from build123d import *

# Parameters (mm, degrees)
SKETCH1_R           = 6
SKETCH1_W           = 9.664317132
SKETCH1_H           = 5.093827802
BOSS_EXTRUDE1_DEPTH = 58
SKETCH2_R           = 2.5
SKETCH2_R_2         = 1.557642262
CUT_EXTRUDE1_DEPTH  = 10


with BuildPart() as part:
    # Sketch1 → Boss-Extrude1 (new body)
    with BuildSketch(Plane.XY):
        with BuildLine():
            Line((-9.822104082, -25.661413332), (-5.082925118, -30.205025059))
            ThreePointArc((-5.082925118, -30.205025059), (-5.444381805, -30.665269108), (-5.771113852, -31.15078089))
            Line((-5.771113852, -31.15078089), (-9.145384533, -28.943772104))
            Line((-9.145384533, -28.943772104), (-9.823578986, -29.980655904))
            Line((-9.823578986, -29.980655904), (-6.344193142, -32.256417352))
            ThreePointArc((-6.344193142, -32.256417352), (-6.488837019, -32.624364602), (-6.615069482, -32.999027645))
            Line((-6.615069482, -32.999027645), (-9.783580045, -32.250497314))
            Line((-9.783580045, -32.250497314), (-10.034391467, -33.312175922))
            Line((-10.034391467, -33.312175922), (-6.865985046, -34.060689065))
            ThreePointArc((-6.865985046, -34.060689065), (-6.932730681, -34.565893765), (-6.967078624, -35.074329589))
            Line((-6.967078624, -35.074329589), (-9.963607891, -35.148687431))
            Line((-9.963607891, -35.148687431), (-9.93976563, -36.109501168))
            Line((-9.93976563, -36.109501168), (-6.926935836, -36.033753282))
            ThreePointArc((-6.926935836, -36.033753282), (-6.847527662, -36.665356301), (-6.717901152, -37.288593816))
            Line((-6.717901152, -37.288593816), (-9.93976563, -37.288593816))
            Line((-9.93976563, -37.288593816), (-9.93976563, -38.42012165))
            Line((-9.93976563, -38.42012165), (-6.362008263, -38.42012165))
            ThreePointArc((-6.362008263, -38.42012165), (-6.149413668, -38.888266643), (-5.907103174, -39.341744119))
            Line((-5.907103174, -39.341744119), (-9.93976563, -39.341744119))
            Line((-9.93976563, -39.341744119), (-9.93976563, -40.709698074))
            Line((-9.93976563, -40.709698074), (-5.907103174, -40.709698074))
            Line((-5.907103174, -40.709698074), (-5.889625491, -41.688448301))
            Line((-5.889625491, -41.688448301), (-9.93976563, -41.688448301))
            Line((-9.93976563, -41.688448301), (-9.93976563, -42.842115912))
            Line((-9.93976563, -42.842115912), (-5.847543839, -42.842115912))
            Line((-5.847543839, -42.842115912), (-5.847543839, -44.079099033))
            Line((-5.847543839, -44.079099033), (-9.93976563, -44.079099033))
            Line((-9.93976563, -44.079099033), (-9.93976563, -45.299533915))
            Line((-9.93976563, -45.299533915), (-5.847543839, -45.299533915))
            Line((-5.847543839, -45.299533915), (-5.847543839, -46.402625605))
            Line((-5.847543839, -46.402625605), (-10.073482588, -46.402625605))
            Line((-10.073482588, -46.402625605), (-10.073482588, -51.367819628))
            Line((-10.073482588, -51.367819628), (-5.904369685, -51.367819628))
            Line((-5.904369685, -51.367819628), (1.003920553, -51.367819628))
            Line((1.003920553, -51.367819628), (7.912210791, -51.367819628))
            Line((7.912210791, -51.367819628), (12.081323694, -51.367819628))
            Line((12.081323694, -51.367819628), (12.081323694, -46.402625605))
            Line((12.081323694, -46.402625605), (7.855384945, -46.402625605))
            Line((7.855384945, -46.402625605), (7.855384945, -45.299533915))
            Line((7.855384945, -45.299533915), (11.947606735, -45.299533915))
            Line((11.947606735, -45.299533915), (11.947606735, -44.079099033))
            Line((11.947606735, -44.079099033), (7.855384945, -44.079099033))
            Line((7.855384945, -44.079099033), (7.855384945, -42.842115912))
            Line((7.855384945, -42.842115912), (11.947606735, -42.842115912))
            Line((11.947606735, -42.842115912), (11.947606735, -41.688448301))
            Line((11.947606735, -41.688448301), (7.897466597, -41.688448301))
            Line((7.897466597, -41.688448301), (7.914944279, -40.709698074))
            Line((7.914944279, -40.709698074), (11.947606735, -40.709698074))
            Line((11.947606735, -40.709698074), (11.947606735, -39.341744119))
            Line((11.947606735, -39.341744119), (7.914944279, -39.341744119))
            ThreePointArc((7.914944279, -39.341744119), (8.157254773, -38.888266643), (8.369849369, -38.42012165))
            Line((8.369849369, -38.42012165), (11.947606735, -38.42012165))
            Line((11.947606735, -38.42012165), (11.947606735, -37.288593816))
            Line((11.947606735, -37.288593816), (8.725742258, -37.288593816))
            ThreePointArc((8.725742258, -37.288593816), (8.855368768, -36.665356301), (8.934776942, -36.033753282))
            Line((8.934776942, -36.033753282), (11.947606735, -36.109501168))
            Line((11.947606735, -36.109501168), (11.971448997, -35.148687431))
            Line((11.971448997, -35.148687431), (8.974919729, -35.074329589))
            ThreePointArc((8.974919729, -35.074329589), (8.940571786, -34.565893765), (8.873826152, -34.060689065))
            Line((8.873826152, -34.060689065), (12.042232573, -33.312175922))
            Line((12.042232573, -33.312175922), (11.791421151, -32.250497314))
            Line((11.791421151, -32.250497314), (8.622910588, -32.999027645))
            ThreePointArc((8.622910588, -32.999027645), (8.496678124, -32.624364602), (8.352034248, -32.256417352))
            Line((8.352034248, -32.256417352), (11.831420091, -29.980655904))
            Line((11.831420091, -29.980655904), (11.153225638, -28.943772104))
            Line((11.153225638, -28.943772104), (7.778954958, -31.15078089))
            ThreePointArc((7.778954958, -31.15078089), (7.452222911, -30.665269108), (7.090766224, -30.205025059))
            Line((7.090766224, -30.205025059), (11.829945188, -25.661413332))
            Line((11.829945188, -25.661413332), (11.155479277, -24.957916896))
            Line((11.155479277, -24.957916896), (6.404976787, -29.512384871))
            ThreePointArc((6.404976787, -29.512384871), (5.847311339, -29.042565295), (5.248984501, -28.625760566))
            Line((5.248984501, -28.625760566), (7.716155949, -25.236928133))
            Line((7.716155949, -25.236928133), (6.917652539, -24.655593749))
            Line((6.917652539, -24.655593749), (4.363311136, -28.164160209))
            ThreePointArc((4.363311136, -28.164160209), (4.135366319, -28.062042381), (3.904321948, -27.967145652))
            Line((3.904321948, -27.967145652), (3.904321948, -24.362789588))
            Line((3.904321948, -24.362789588), (-1.896480842, -24.362789588))
            Line((-1.896480842, -24.362789588), (-1.896480842, -27.967145652))
            ThreePointArc((-1.896480842, -27.967145652), (-2.127525214, -28.062042381), (-2.35547003, -28.164160209))
            Line((-2.35547003, -28.164160209), (-4.909811434, -24.655593749))
            Line((-4.909811434, -24.655593749), (-5.708314844, -25.236928133))
            Line((-5.708314844, -25.236928133), (-3.241143396, -28.625760566))
            ThreePointArc((-3.241143396, -28.625760566), (-3.839470233, -29.042565295), (-4.397135681, -29.512384871))
            Line((-4.397135681, -29.512384871), (-9.147638171, -24.957916896))
            Line((-9.147638171, -24.957916896), (-9.822104082, -25.661413332))
        make_face()
        with Locations((1.003920553, -35.357441113)):
            Circle(SKETCH1_R, mode=Mode.SUBTRACT)
        with Locations((0.899494134, -46.834148598)):
            Rectangle(SKETCH1_W, SKETCH1_H, mode=Mode.SUBTRACT)
    extrude(amount=BOSS_EXTRUDE1_DEPTH)

    # Sketch2 → Cut-Extrude1 (cut)
    with BuildSketch(Plane.XZ.offset(51.367819628)):
        with Locations((1.188364706, 29)):
            Circle(SKETCH2_R)
        with Locations((-6.573482588, 10)):
            Circle(SKETCH2_R_2)
        with Locations((9.191259736, 10.100266019)):
            Circle(SKETCH2_R_2)
        with Locations((9.191259736, 47.899733981)):
            Circle(SKETCH2_R_2)
        with Locations((-6.573482588, 48)):
            Circle(SKETCH2_R_2)
    extrude(amount=-CUT_EXTRUDE1_DEPTH, mode=Mode.SUBTRACT)


solid = part.part
Can you work these out from the model? Positions are in its coordinate system, mm. A direction names the side the tool comes from. Coordinates: 2 decimals unless noted, no trailing zeros. Write each loop counter-clockwise with the first axis right and the second up, starting at its lowest first coordinate (ties: lowest second). Pieces come first, ordered by that corner, then holes. Notation, with made-up numbers: (-11.5, 78) - (35.5, 78) arc R20 ccw to (35.5, 100) - close; hole circle Ø2 at (-1.5, 68.25). An arc over 180 degrees is marked (long way). Return JSON: item names as keys, results as strings. Group by question number.
Item 1: Please list where these lines run through material, in increasing order: probe 1 along Y at (x, z) = (-4.5, 43.5); probe 2 along Y at (x, z) = (5.5, 5); probe 3 along X at (y, z) = (-28.5, 19).
Item 2: If we section it at B-B (z = 13.5): Count the separate pieces of the cut face and the enclosed holes in it, then the cut area to 3 significant figures.
Item 3: We'd pull the mould along X, two halves only. Please class faces 5 (the face through (-2, -44.287, 29)), 6 (the face through (10, -44.079, 29)), 7 (the face through (-9.48, -29.455, 28.594)): pulls with the +X half, pulls with the -X half, needs draft (parallel to the pull), parting line crosses it, or undercut.
Item 4: Which directions (+Z, -Z, +X, -X, +Y, -Y) give clear straight access to the entire face, cutting with the end or side of a thin tool? Please do faces 1 (the face through (7.635, -46.438, 47.968)), 2 (the face through (10, -42.842, 29)), 3 (the face through (-8, -41.688, 29)), 4 (the face through (-7.435, -30.063, 28.594)).
Item 5: I'm going to push flat-ended pins straight in: pin 1 Ø0.7 at (x, z) = (-5.5, 10) entering from -Y; pin 2 Ø2 at (x, z) = (7, 33) entering from +Y; pin 3 Ø2 at (x, z) = (10.5, 39.5) entering from +Y. Where does each tip first touch, or does it pass through?
Item 6: If we section it at A-A (x = 2.5): Write out the boundary of the cut face in (y, z).
Return value:
{
 "1": {"probe 1": "y = -51.37 to -37.75, -32.97 to -29.41, -26.9 to -25.22", "probe 2": "y = -51.37 to -49.38, -44.29 to -39.33, -31.38 to -28.79, -28.28 to -26.6", "probe 3": "x = -6.86 to -5.45, -3.33 to 5.34, 7.46 to 8.87"},
 "2": {"separate pieces": "1", "enclosed holes": "2", "area": "306 mm^2"},
 "3": {"face 5": "undercut", "face 6": "needs draft", "face 7": "pulls with the -X half"},
 "4": {"face 1": "-Y", "face 2": "+Z, -Z, +X", "face 3": "+Z, -Z, -X", "face 4": "+Z, -Z"},
 "5": {"pin 1": "stops at y = -41.37", "pin 2": "stops at y = -24.66", "pin 3": "stops at y = -24.96"},
 "6": {"outline": "(-51.37, 0) - (-49.38, 0) - (-49.38, 26.87) - (-51.37, 26.87) - close; (-51.37, 31.13) - (-49.38, 31.13) - (-49.38, 58) - (-51.37, 58) - close; (-44.29, 0) - (-41.17, 0) - (-41.17, 58) - (-44.29, 58) - (-44.29, 31.13) - (-41.37, 31.13) - (-41.37, 26.87) - (-44.29, 26.87) - close; (-29.55, 0) - (-24.36, 0) - (-24.36, 58) - (-29.55, 58) - close"}
}
